```python
from build123d import *

# Parameters (mm, degrees)
F0_R     = 25.4
F0_R_2   = 8.89
F1_DEPTH = 2.54
F2_R     = 25.4
F2_R_2   = 8.89
F3_DEPTH = 20.32
F4_R     = 5.08


with BuildPart() as f1:
    # F0 (on Top) → F1 (new body)
    with BuildSketch(Plane.XY):
        Circle(F0_R)
        Circle(F0_R_2, mode=Mode.SUBTRACT)
    extrude(amount=F1_DEPTH)

    # F2 (on face) → F3 (join)
    with BuildSketch(Plane.XY.offset(2.54)):
        Circle(F2_R)
        Circle(F2_R_2, mode=Mode.SUBTRACT)
        Circle(F2_R_2)
    extrude(amount=F3_DEPTH)

    # F4
    f4_edges = [f1.edges().sort_by_distance(p)[0] for p in [
        (-25.4, 0, 22.86),
    ]]
    fillet(f4_edges, radius=F4_R)


solid = f1.part
```
Design review of the part built by this model. Coordinates are the model's own, in mm. A direction names the side the tool comes from. Give positions to 0.01 mm unless a question says otherwise; leave off trailing zeros. Order: outer loops, then holes, each group sorted by start corner. A loop starts at its lowest first (then second) coordinate and runs counter-clockwise, first axis right, second up. Notation, with made-up numbers: (-2.5, -14) -> (40.5, -14) arc R27 cw to (40.5, 17) -> close; hole circle Ø1 at (12.25, 59). An arc over 180 degrees is marked (long way). Write item = value, one per line. Start each with the question number.
(1) We need section A-A on x = 0. Write out the cut boundary in (y, z), plus the area to 3 significant figures.
(2) For faces 4 (the face through (-1.93, -8.68, 1.25)), 5 (the face through (11, 0, 0)), list the 3-axis set-ups (+Z, -Z, +X, -X, +Y, -Y) from which the entire face can be reached by the end or side of a thin tool; tool diameter is ignored.
(3) Mouldability with a two-part tool opening along Y and no side actions: class faces 1 (the face through (-5.506, -24.796, 8.766)), 2 (the face through (0, 0, 2.54)), 3 (the face through (0, 0, 22.86)) as +Y half, -Y half, draft (parallel to the pull), parting line (faces both ways), or undercut.
(4) For pin 1 (3 mm diameter, centred on y = -12, z = 15, fed in from +X); pin 2 (5 mm diameter, centred on y = 15, z = 3, fed in from -X); pin 3 (1.5 mm diameter, centred on y = 12, z = 5.5, fed in from +X), all flat-tipped, find the tip position at first contact; note any pin that passes through.
(5) We need section C-C on z = 11. Write out the cut boundary in (x, y), plus the area to 3 significant figures.
(6) To check wall thickness, follow line 1 along Y through (x, z) = (0, 0.5); line 2 along Z through (x, y) = (-16.5, -12); line 3 along X through (y, z) = (-1.5, 9.5). State the ranges of each line that lie inside material, in increasing order.
Numbers:
q1.outline = (-25.4, 0) -> (-8.89, 0) -> (-8.89, 2.54) -> (8.89, 2.54) -> (8.89, 0) -> (25.4, 0) -> (25.4, 17.78) arc R5.08 ccw to (20.32, 22.86) -> (-20.32, 22.86) arc R5.08 ccw to (-25.4, 17.78) -> close
q1.area = 1,110 mm^2
q2.face_4 = -Z
q2.face_5 = -Z, +X, -X, +Y, -Y
q3.face_1 = parting line
q3.face_2 = undercut
q3.face_3 = draft
q4.pin_1 = 23.13
q4.pin_2 = -22.11
q4.pin_3 = 22.77
q5.outline = circle Ø50.8 at (0, 0)
q5.area = 2,030 mm^2
q6.line_1 = -25.4 to -8.89, 8.89 to 25.4
q6.line_2 = 0 to 22.86
q6.line_3 = -25.36 to 25.36
